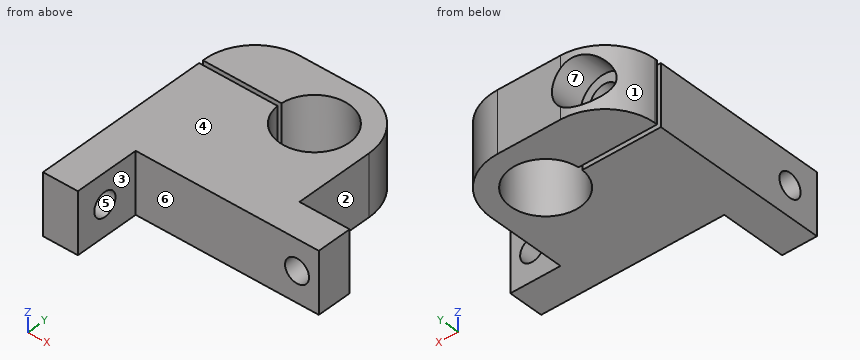
from build123d import *

# Parameters (mm, degrees)
EXTRUDE_1_DEPTH               = 14
SKETCH_2_R                    = 2.75
CUT_EXTRUDE_1_DEPTH           = 49.520614176
SKETCH_3_R                    = 2.75
CUT_EXTRUDE_2_DEPTH           = 67.158899628
HOLE_START                    = 5.1
HOLE_WIZARD_M61_OUTLINE_R     = 5.5
HOLE_WIZARD_M61_DEPTH         = 7.4
HOLE_START_2                  = 0.5
HOLE_WIZARD_M61_2_OUTLINE_R   = 3.3
HOLE_WIZARD_M61_2_DEPTH       = 4.6
HOLE_WIZARD_M61_3_D           = 5
HOLE_WIZARD_M61_3_DEPTH       = 17
HOLE_WIZARD_M61_3_CSINK_D     = 6.05
HOLE_WIZARD_M61_3_CSINK_ANGLE = 120
HOLE_WIZARD_M61_3_TIP         = 1.502151548


# Read off the part's stored shape, not the designer's step: Цековка для  винта с внутренним шестигранником M61
with BuildPart() as part:
    # Эскиз1 → Бобышка-Вытянуть1 (new body)
    with BuildSketch(Plane.XY):
        with BuildLine():
            Line((-26, 0.5), (-7.984359711, 0.5))
            ThreePointArc((-7.984359711, 0.5), (8, 0), (-7.984359711, -0.5))
            Line((-7.984359711, -0.5), (-26, -0.5))
            Line((-26, -0.5), (-26, -18))
            Line((-26, -18), (-26, -26))
            Line((-26, -26), (-26, -41))
            Line((-26, -41), (-18, -41))
            Line((-18, -41), (-18, -26))
            Line((-18, -26), (24, -26))
            Line((24, -26), (24, -18))
            Line((24, -18), (12.5, -18))
            Line((12.5, -18), (12.5, 0))
            ThreePointArc((12.5, 0), (8.838834765, 8.838834765), (0, 12.5))
            Line((0, 12.5), (-14.5, 12.5))
            ThreePointArc((-14.5, 12.5), (-22.631727984, 9.131727984), (-26, 1))
            Line((-26, 1), (-26, 0.5))
        make_face()
    extrude(amount=EXTRUDE_1_DEPTH)

    # Эскиз2 → Вырез-Вытянуть1 (cut, through all)
    with BuildSketch(Plane.XZ.offset(26)):
        with Locations(Location((19, 7, 0), (0, 0, 270))):
            Circle(SKETCH_2_R)
    extrude(amount=-CUT_EXTRUDE_1_DEPTH, mode=Mode.SUBTRACT)

    # Эскиз3 → Вырез-Вытянуть2 (cut, through all)
    with BuildSketch(Plane.ZY.offset(26)):
        with Locations((7, -34)):
            Circle(SKETCH_3_R)
    extrude(amount=-CUT_EXTRUDE_2_DEPTH, mode=Mode.SUBTRACT)

    # Hole Wizard M61 outline → Hole Wizard M61 (cut)
    with BuildSketch(Plane(origin=(0, 0, 0), x_dir=(1, 0, 0), z_dir=(0, 1, 0)).offset(HOLE_START)):
        with Locations((-18, -7)):
            Circle(HOLE_WIZARD_M61_OUTLINE_R)
    extrude(amount=HOLE_WIZARD_M61_DEPTH, mode=Mode.SUBTRACT)

    # Hole Wizard M61 2 outline → Hole Wizard M61 2 (cut)
    with BuildSketch(Plane(origin=(0, 0, 0), x_dir=(1, 0, 0), z_dir=(0, 1, 0)).offset(HOLE_START_2)):
        with Locations((-18, -7)):
            Circle(HOLE_WIZARD_M61_2_OUTLINE_R)
    extrude(amount=HOLE_WIZARD_M61_2_DEPTH, mode=Mode.SUBTRACT)

    # Hole Wizard M61 3
    with Locations(Plane(origin=(0, -0.5, 0), x_dir=(-1, 0, 0), z_dir=(0, 1, 0))):
        with Locations((18, 7)):
            CounterSinkHole(HOLE_WIZARD_M61_3_D / 2, HOLE_WIZARD_M61_3_CSINK_D / 2, depth=HOLE_WIZARD_M61_3_DEPTH, counter_sink_angle=HOLE_WIZARD_M61_3_CSINK_ANGLE)
            with Locations((0, 0, -(HOLE_WIZARD_M61_3_DEPTH + HOLE_WIZARD_M61_3_TIP / 2))):  # 118° drill point
                Cone(0, HOLE_WIZARD_M61_3_D / 2, HOLE_WIZARD_M61_3_TIP, mode=Mode.SUBTRACT)


solid = part.part
The listing builds one solid part. Answer for the finished solid, in the listing's coordinates (mm). Face numbers are marked on the shaded views. A direction names the side the tool comes from. Coordinates: 2 decimals unless noted, no trailing zeros. Write each loop counter-clockwise with the first axis right and the second up, starting at its lowest first coordinate (ties: lowest second). Pieces come first, ordered by that corner, then holes. Notation, with made-up numbers: (68.25, 24) - (76.25, 24) arc R20 cw to (76.25, 61) - close; hole circle Ø6 at (48, 37.25). An arc over 180 degrees is marked (long way). Return JSON: item names as keys, results as strings.
1. The part is cut by section A-A on x = 19. Determine the outline of the cut face in (y, z).
Final values:
{"outline": "(-26, 0) - (-18, 0) - (-18, 4.25) - (-26, 4.25) - close; (-26, 9.75) - (-18, 9.75) - (-18, 14) - (-26, 14) - close"}
2. The part is cut by section C-C on y = -24. Determine the outline of the cut face in (x, z).
Final values:
{"outline": "(-26, 0) - (24, 0) - (24, 14) - (-26, 14) - close; hole circle Ø5.5 at (19, 7)"}
3. Which of the six approach directions +Z, -Z, +X, -X, +Y, -Y give full straight-line access (tool end or side, diameter ignored) to the marked faces 1, 2 and 3?
Final values:
{"face 1": "+Z, -Z, -X, +Y", "face 2": "+Z, -Z, +X, +Y", "face 3": "+Z, -Z, +X, -Y"}
4. The part is cut by section B-B on y = 4.5. Determine the outline of the cut face in (x, z), then the cut area to 3 significant figures.
Final values:
{"outline": "(-25.45, 0) - (-6.61, 0) - (-6.61, 14) - (-25.45, 14) - close; (6.61, 0) - (11.66, 0) - (11.66, 14) - (6.61, 14) - close; hole circle Ø6.6 at (-18, 7)", "area": "300 mm^2"}
5. The part is cut by section D-D on x = -7. Determine the outline of the cut face in (y, z), then the cut area to 3 significant figures.
Final values:
{"outline": "(-26, 0) - (-3.87, 0) - (-3.87, 14) - (-26, 14) - close; (3.87, 0) - (12.5, 0) - (12.5, 14) - (3.87, 14) - close", "area": "431 mm^2"}
6. Consider line 1 along Z through (x, y) = (-18, 2); line 2 along Z through (x, y) = (-18, -9.75); line 3 along Y through (x, z) = (-16.5, 3.5). Determine where each line is inside the solid, lowest interval first.
Final values:
{"line 1": "0 to 3.7, 10.3 to 14", "line 2": "0 to 4.5, 9.5 to 14", "line 3": "-26 to -0.5, 0.5 to 5.1"}
7. Each of these flat-tipped pins is pushed along its axis until it touches: pin 1 Ø18.5 at (x, y) = (0, 0) entering from -Z; pin 2 Ø6 at (x, z) = (18.5, 10) entering from +Y; pin 3 Ø5 at (x, z) = (5, 9.5) entering from -Y; pin 4 Ø4 at (y, z) = (-33, 4) entering from +X. Where does it stop, or does it pass through?
Final values:
{"pin 1": "z = 0", "pin 2": "y = -18", "pin 3": "y = -26", "pin 4": "x = -18"}
8. For a pull along Z with two mould halves and no side action, classify the marked faces 4, 5, 6 and 7 as +Z half, -Z half, draft (parallel to the pull), parting line (faces both ways), or undercut.
Final values:
{"face 4": "+Z half", "face 5": "undercut", "face 6": "draft", "face 7": "undercut"}
